CAD build for the part. Positions are in the model's coordinates, mm. A direction names the side the tool comes from. Give positions to 0.01 mm unless a question says otherwise; leave off trailing zeros. Put each result on its own line as item: value. Start each with the question number.
1) Two-plate mould, pull along X, no slides. Class faces 1 (the face through (-393, -17, 0)), 2 (the face through (-304, -17, 1.588)): released by +X, released by -X, zero draft, split by the parting line, or undercut.
2) Pin check, flat tips, straight feed: pin 1 (2 mm diameter, centred on y = 508.5, z = 6.5, fed in from -X); pin 2 (6 mm diameter, centred on x = 255.5, y = 606, fed in from +Z); pin 3 (9.5 mm diameter, centred on x = 360, y = 350.5, fed in from -Z). Stop position of each tip, or through.
3) Drill centre lines: line 1 (X direction, y = -387.5, z = 13.5); line 2 (X direction, y = -469.5, z = 18); line 3 (Z direction, x = -50, y = 289). Where is each one in solid material? Low to high. Write a range as [from, to].
4) Tool access for faces 3 (the face through (393, -17, 0)), 4 (the face through (0, -17, 1.588)): list every direction of +Z, -Z, +X, -X, +Y, -Y with a clear straight run to the whole face (end or side of a thin tool).
```python
from build123d import *

# Parameters (mm, degrees)
F1_DEPTH = 1219.2


with BuildPart() as f1:
    # F0 (on Front) → F1 (new body, symmetric)
    with BuildSketch(Plane.XZ):
        Polygon((-33.3375, 0), (33.3375, 0), (41.275, 4.7625), (60.325, 4.7625), (68.2625, 0), (107.95, 0), (139.7, 31.75), (165.1, 31.75), (196.85, 0), (236.5375, 0), (244.475, 4.7625), (263.525, 4.7625), (271.4625, 0), (338.1375, 0), (346.075, 4.7625), (365.125, 4.7625), (373.0625, 0), (412.75, 0), (444.5, 31.75), (469.9, 31.75), (482.6, 19.05), (483.722532, 20.172532), (470.557564, 33.3375), (443.842436, 33.3375), (412.092436, 1.5875), (373.502212, 1.5875), (365.564712, 6.35), (345.635288, 6.35), (337.697788, 1.5875), (271.902212, 1.5875), (263.964712, 6.35), (244.035288, 6.35), (236.097788, 1.5875), (197.507564, 1.5875), (165.757564, 33.3375), (139.042436, 33.3375), (107.292436, 1.5875), (68.702212, 1.5875), (60.764712, 6.35), (40.835288, 6.35), (32.897788, 1.5875), (-32.897788, 1.5875), (-40.835288, 6.35), (-60.764712, 6.35), (-68.702212, 1.5875), (-107.292436, 1.5875), (-139.042436, 33.3375), (-165.757564, 33.3375), (-197.507564, 1.5875), (-236.097788, 1.5875), (-244.035288, 6.35), (-263.964712, 6.35), (-271.902212, 1.5875), (-337.697788, 1.5875), (-345.635288, 6.35), (-365.564712, 6.35), (-373.502212, 1.5875), (-412.092436, 1.5875), (-443.842436, 33.3375), (-470.557564, 33.3375), (-483.722532, 20.172532), (-482.6, 19.05), (-469.9, 31.75), (-444.5, 31.75), (-412.75, 0), (-373.0625, 0), (-365.125, 4.7625), (-346.075, 4.7625), (-338.1375, 0), (-271.4625, 0), (-263.525, 4.7625), (-244.475, 4.7625), (-236.5375, 0), (-196.85, 0), (-165.1, 31.75), (-139.7, 31.75), (-107.95, 0), (-68.2625, 0), (-60.325, 4.7625), (-41.275, 4.7625), align=None)
    extrude(amount=F1_DEPTH, both=True)


solid = f1.part
```
Solution:
1. face 1: zero draft
1. face 2: undercut
2. pin 1: x = -420.25
2. pin 2: z = 6.35
2. pin 3: z = 4.76
3. line 1: [-426.25, -424], [-185.6, -183.35], [-121.45, -119.2], [119.2, 121.45], [183.35, 185.6], [424, 426.25]
3. line 2: [-430.75, -428.5], [-181.1, -178.85], [-125.95, -123.7], [123.7, 125.95], [178.85, 181.1], [428.5, 430.75]
3. line 3: [4.76, 6.35]
4. face 3: -Z, +X, -X, +Y, -Y
4. face 4: +Z, +Y, -Y
